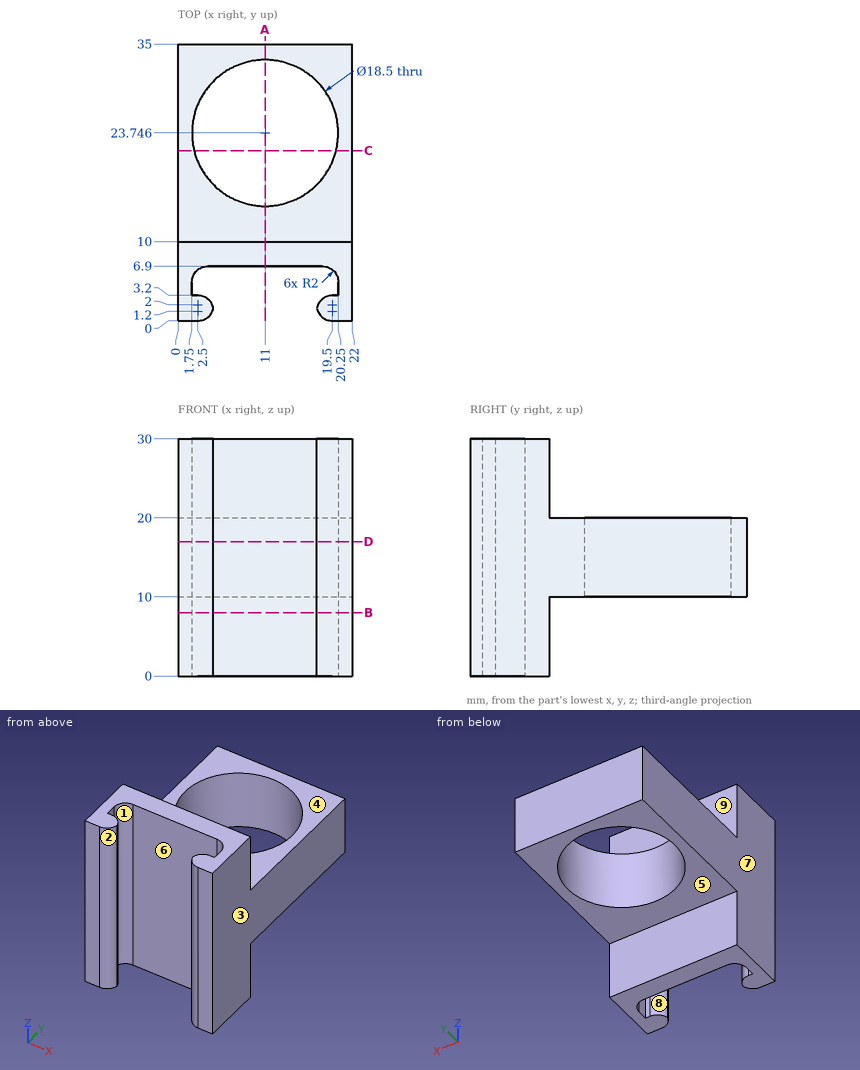
Print and shaded views of the part. All mm, measured from the part's lowest x, y and z. A direction names the side the tool comes from. Coordinates: 2 decimals unless noted, no trailing zeros. Order: outer loops, then holes, each group sorted by start corner. A loop starts at its lowest first (then second) coordinate and runs counter-clockwise, first axis right, second up.
Item 1: Saw through at B-B on z = 8. List the corners of the cut face in (x, y).
Filled in:
outline: (0, 0) - (2.5, 0) arc R2 ccw to (4.46, 1.6) arc R2 ccw to (2.5, 3.2) - (1.75, 3.2) - (1.75, 4.9) arc R2 cw to (3.75, 6.9) - (18.25, 6.9) arc R2 cw to (20.25, 4.9) - (20.25, 3.2) - (19.5, 3.2) arc R2 ccw to (17.54, 1.6) arc R2 ccw to (19.5, 0) - (22, 0) - (22, 10) - (0, 10) - close
Item 2: Tool access for the marked faces 1, 2, 3, 4 and 5: list every direction of +Z, -Z, +X, -X, +Y, -Y with a clear straight run to the whole face (end or side of a thin tool).
Filled in:
face 1: +Z, -Z
face 2: +Z, -Z, -Y
face 3: +Z, -Z, +X, +Y, -Y
face 4: +Z, +X, -X, +Y
face 5: -Z, +X, -X, +Y
Item 3: Saw through at A-A on x = 11. List the corners of the cut face in (y, z), then the cut area to 3 significant figures.
Filled in:
outline: (6.9, 0) - (10, 0) - (10, 10) - (14.5, 10) - (14.5, 20) - (10, 20) - (10, 30) - (6.9, 30) - close; (33, 10) - (35, 10) - (35, 20) - (33, 20) - close
area: 158 mm2
Item 4: Saw through at D-D on z = 17. List the corners of the cut face in (x, y), then the cut area to 3 significant figures.
Filled in:
outline: (0, 0) - (2.5, 0) arc R2 ccw to (4.46, 1.6) arc R2 ccw to (2.5, 3.2) - (1.75, 3.2) - (1.75, 4.9) arc R2 cw to (3.75, 6.9) - (18.25, 6.9) arc R2 cw to (20.25, 4.9) - (20.25, 3.2) - (19.5, 3.2) arc R2 ccw to (17.54, 1.6) arc R2 ccw to (19.5, 0) - (22, 0) - (22, 35) - (0, 35) - close; hole circle Ø18.5 at (11, 23.75)
area: 389 mm2
Item 5: Drill centre lines: L1, parallel to Y at x = 11, z = 15; L2, parallel to Y at x = 14.25, z = 12.75; L3, parallel to Z at x = 19, y = 16. Where is each one in solid material? Low to high.
Filled in:
L1: y = 6.9 to 14.5, 33 to 35
L2: y = 6.9 to 15.09, 32.41 to 35
L3: z = 10 to 20
Item 6: Drop flat-ended pins along their axis: pin 1 Ø3 at (x, z) = (14, 11) entering from -Y; pin 2 Ø8 at (x, z) = (6.5, 6.5) entering from +Y; pin 3 Ø7 at (x, z) = (7.5, 22.5) entering from -Y; pin 4 Ø8 at (x, y) = (12.5, 16.5) entering from +Z. Give the stop position or say it passes through.
Filled in:
pin 1: stops at y = 6.9
pin 2: stops at y = 35
pin 3: stops at y = 0.68
pin 4: stops at z = 20
Item 7: Mould opens along X. For the marked faces 6, 7, 8 and 9 say: released by +X, released by -X, zero draft, split by the parting line, or undercut.
Filled in:
face 6: undercut
face 7: released by -X
face 8: undercut
face 9: zero draft
Item 8: Saw through at C-C on y = 21.5. List the corners of the cut face in (x, z), then the cut area to 3 significant figures.
Filled in:
outline: (0, 10) - (2.03, 10) - (2.03, 20) - (0, 20) - close; (19.97, 10) - (22, 10) - (22, 20) - (19.97, 20) - close
area: 40.5 mm2
